Can you work these out from the drawing? Everything is in mm from the part's minimum corner. A direction names the side the tool comes from. Coordinates: 2 decimals unless noted, no trailing zeros. Loops run counter-clockwise (first coordinate to the right, second up) from the corner with the lowest first, then second, coordinate; pieces in that order, holes last. Notation, with made-up numbers: (85, 68) -> (115, 68) arc R18 ccw to (115, 90) -> close; hole circle Ø4 at (-29, 56). An arc over 180 degrees is marked (long way). Put each result on its own line as item: value. Start each with the question number.
Item 1: For the marked faces 5 and 6, which set-ups out of +Z, -Z, +X, -X, +Y, -Y let a thin tool reach every point of the face, with its end or its side?
Item 2: If we section it at A-A on y = 12.7: Please give me the cut outline in (x, z), plus the area to 3 significant figures.
Item 3: If we section it at B-B on x = 38.1: Please give me the cut outline in (y, z).
Item 4: Will these pins go through, and if not, where does the flat tip stop? P1, Ø3, axis at x = 54.5, y = 21, coming from the -Z side; P2, Ø1.9, axis at y = 15.5, z = 16.5, coming from the +X side; P3, Ø2, axis at x = 15.5, z = 17, coming from the -Y side; P4, Ø3, axis at x = 3, y = 18, coming from the +Z side.
Item 5: Please list where these lines run through material, in increasing order: L1, parallel to X at y = 8.25, z = 14.75; L2, parallel to Y at x = 38.1, z = 8.25; L3, parallel to Z at x = 43.5, y = 18.75. Write a range as from..to.
Item 6: We'd pull the mould along X, two halves only. Please class the marked faces 1, 2, 3 and 4: pulls with the +X half, pulls with the -X half, needs draft (parallel to the pull), parting line crosses it, or undercut.
Item 7: If we section it at C-C on z = 15.25: Please give me the cut outline in (x, y).
Item 8: If we section it at D-D on y = 9.75: Please give me the cut outline in (x, z).
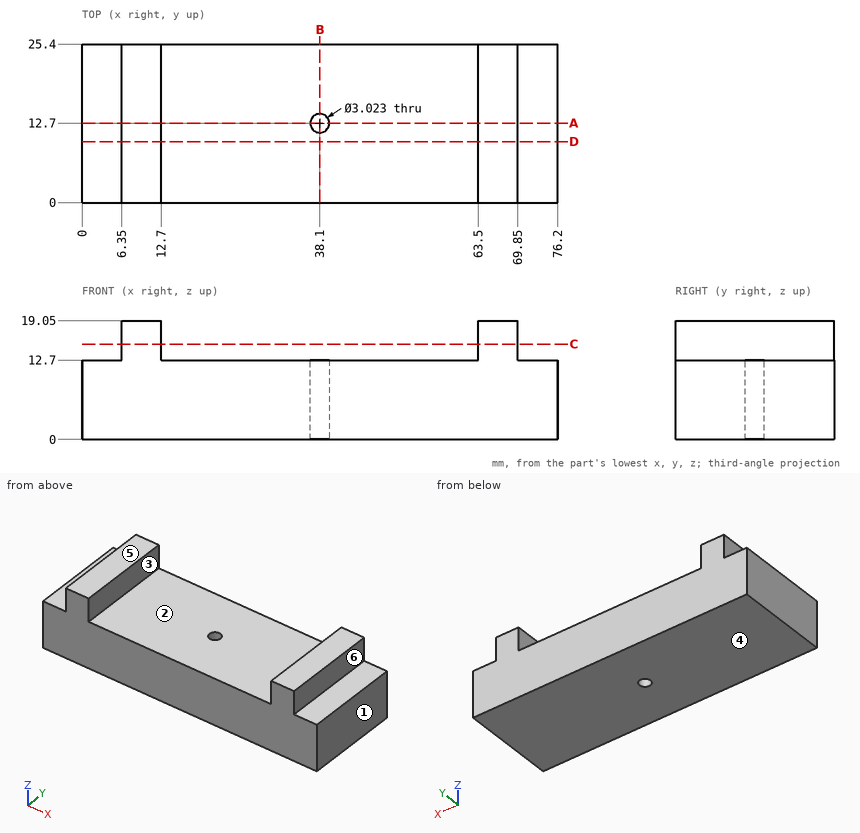
Solutions:
1. face 5: +Z, +X, -X, +Y, -Y
1. face 6: +Z, +X, +Y, -Y
2. outline: (0, 0) -> (36.59, 0) -> (36.59, 12.7) -> (12.7, 12.7) -> (12.7, 19.05) -> (6.35, 19.05) -> (6.35, 12.7) -> (0, 12.7) -> close; (39.61, 0) -> (76.2, 0) -> (76.2, 12.7) -> (69.85, 12.7) -> (69.85, 19.05) -> (63.5, 19.05) -> (63.5, 12.7) -> (39.61, 12.7) -> close
2. area: 1,010 mm^2
3. outline: (0, 0) -> (11.19, 0) -> (11.19, 12.7) -> (0, 12.7) -> close; (14.21, 0) -> (25.4, 0) -> (25.4, 12.7) -> (14.21, 12.7) -> close
4. P1: z = 0
4. P2: x = 69.85
4. P3: through
4. P4: z = 12.7
5. L1: 6.35..12.7, 63.5..69.85
5. L2: 0..11.19, 14.21..25.4
5. L3: 0..12.7
6. face 1: pulls with the +X half
6. face 2: undercut
6. face 3: undercut
6. face 4: needs draft
7. outline: (6.35, 0) -> (12.7, 0) -> (12.7, 25.4) -> (6.35, 25.4) -> close; (63.5, 0) -> (69.85, 0) -> (69.85, 25.4) -> (63.5, 25.4) -> close
8. outline: (0, 0) -> (76.2, 0) -> (76.2, 12.7) -> (69.85, 12.7) -> (69.85, 19.05) -> (63.5, 19.05) -> (63.5, 12.7) -> (12.7, 12.7) -> (12.7, 19.05) -> (6.35, 19.05) -> (6.35, 12.7) -> (0, 12.7) -> close
